```python
from build123d import *

# Parameters (mm, degrees)
SKETCH_1_R      = 1.5
EXTRUDE_1_DEPTH = 60
SKETCH_2_R      = 11
EXTRUDE_2_DEPTH = 2
SKETCH_3_R      = 2.5
EXTRUDE_3_DEPTH = 22


with BuildPart() as part:
    # 草圖1 → 填料-伸長1 (new body)
    with BuildSketch(Plane(origin=(0, 0, 0), x_dir=(1, 0, 0), z_dir=(0, 1, 0))):
        Polygon((-15.5, 21.15), (15.5, 21.15), (21.15, 15.5), (21.15, -15.5), (15.5, -21.15), (-15.5, -21.15), (-21.15, -15.5), (-21.15, 15.5), align=None)
        with Locations(Location((-15.5, 15.5, 0), (0, 0, 90))):
            Circle(SKETCH_1_R, mode=Mode.SUBTRACT)
        with Locations(Location((15.5, 15.5, 0), (0, 0, 90))):
            Circle(SKETCH_1_R, mode=Mode.SUBTRACT)
        with Locations(Location((15.5, -15.5, 0), (0, 0, 90))):
            Circle(SKETCH_1_R, mode=Mode.SUBTRACT)
        with Locations(Location((-15.5, -15.5, 0), (0, 0, 90))):
            Circle(SKETCH_1_R, mode=Mode.SUBTRACT)
    extrude(amount=EXTRUDE_1_DEPTH)

    # 草圖2 → 填料-伸長2 (add)
    with BuildSketch(Plane(origin=(0, 60, 0), x_dir=(1, 0, 0), z_dir=(0, 1, 0))):
        with Locations(Location((0, 0, 0), (0, 0, 90))):
            Circle(SKETCH_2_R)
    extrude(amount=EXTRUDE_2_DEPTH)

    # 草圖3 → 填料-伸長3 (add)
    with BuildSketch(Plane(origin=(0, 62, 0), x_dir=(1, 0, 0), z_dir=(0, 1, 0))):
        with Locations(Location((0, 0, 0), (0, 0, 270))):
            Circle(SKETCH_3_R)
    extrude(amount=EXTRUDE_3_DEPTH)


solid = part.part
```
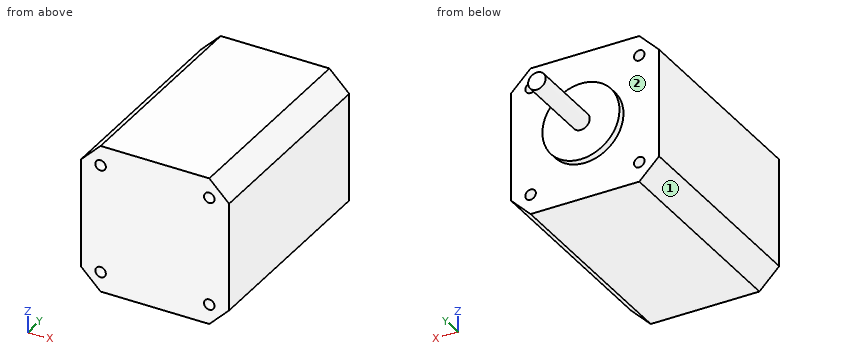
Check sheet for the modelled part. Datum: model origin and axes. Units: mm. Face numbers are marked on the shaded views. A direction names the side the tool comes from. Round coordinates to 2 decimals unless told otherwise and drop trailing zeros. Write each loop counter-clockwise with the first axis right and the second up, starting at its lowest first coordinate (ties: lowest second). Pieces come first, ordered by that corner, then holes. Notation, with made-up numbers: (79.5, -17.5) -> (84.5, -17.5) arc R37 ccw to (84.5, 18.5) -> close; hole circle Ø8 at (84.25, -0.5). An arc over 180 degrees is marked (long way). Put each result on its own line as item: value.
(1) Sectioned sample at B-B (x = 0). Enter the section's corners in (y, z).
Values found:
outline: (0, -21.15) -> (60, -21.15) -> (60, -11) -> (62, -11) -> (62, -2.5) -> (84, -2.5) -> (84, 2.5) -> (62, 2.5) -> (62, 11) -> (60, 11) -> (60, 21.15) -> (0, 21.15) -> close
(2) Go/stop test with flat-tipped pins: pin 1 Ø8 at (x, z) = (-7, -8.5) entering from +Y; pin 2 Ø6 at (x, z) = (-11, 12.5) entering from +Y. Record where each tip stops, or that it passes through.
Values found:
pin 1: stops at y = 62
pin 2: stops at y = 60
(3) Sectioned sample at D-D (x = -6). Enter the section's corners in (y, z).
Values found:
outline: (0, -21.15) -> (60, -21.15) -> (60, -9.22) -> (62, -9.22) -> (62, 9.22) -> (60, 9.22) -> (60, 21.15) -> (0, 21.15) -> close
(4) Sectioned sample at A-A (y = 33.5). Enter the section's corners in (x, z).
Values found:
outline: (-21.15, -15.5) -> (-15.5, -21.15) -> (15.5, -21.15) -> (21.15, -15.5) -> (21.15, 15.5) -> (15.5, 21.15) -> (-15.5, 21.15) -> (-21.15, 15.5) -> close; hole circle Ø3 at (-15.5, -15.5); hole circle Ø3 at (-15.5, 15.5); hole circle Ø3 at (15.5, -15.5); hole circle Ø3 at (15.5, 15.5)
(5) Sectioned sample at C-C (z = 0). Enter the section's corners in (x, y), plus the area to 3 significant figures.
Values found:
outline: (-21.15, 0) -> (21.15, 0) -> (21.15, 60) -> (11, 60) -> (11, 62) -> (2.5, 62) -> (2.5, 84) -> (-2.5, 84) -> (-2.5, 62) -> (-11, 62) -> (-11, 60) -> (-21.15, 60) -> close
area: 2,690 mm^2
(6) Material ranges on line 1 (Z direction, x = -15.5, y = 18); line 2 (X direction, y = 18, z = -15), recorded low to high.
Values found:
line 1: z = -21.15 to -17, -14 to 14, 17 to 21.15
line 2: x = -21.15 to -16.91, -14.09 to 14.09, 16.91 to 21.15
(7) Tool access check on the marked faces 1 and 2. Record the directions out of +Z, -Z, +X, -X, +Y, -Y that give a thin tool (end or side, any length) a straight path to the whole face; none if there is none.
Values found:
face 1: -Z, -X, +Y, -Y
face 2: +Y
